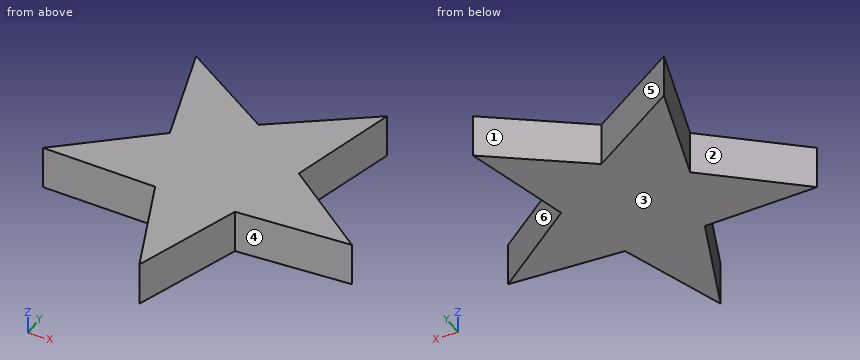
```python
from build123d import *

# Parameters (mm, degrees)
F1_DEPTH = 2


with BuildPart() as f1:
    # F0 (on Top) → F1 (new body)
    with BuildSketch(Plane.XY):
        Polygon((-2.938926, 0.954915), (0, 3.09017), (-4.349611, 5.986726), align=None)
        Polygon((4.349611, 5.986726), (0, 3.09017), (2.938926, 0.954915), align=None)
        Polygon((2.938926, 0.954915), (0, 3.09017), (-2.938926, 0.954915), (-1.816356, -2.5), (0, -2.5), (1.816356, -2.5), align=None)
        Polygon((-1.816356, -2.5), (-2.938926, 0.954915), (-7.037818, -2.286726), align=None)
        Polygon((0, -2.5), (-1.816356, -2.5), (0, -7.4), align=None)
        Polygon((7.037818, -2.286726), (2.938926, 0.954915), (1.816356, -2.5), align=None)
        Polygon((0, -7.4), (1.816356, -2.5), (0, -2.5), align=None)
    extrude(amount=F1_DEPTH)


solid = f1.part
```
Work out the finished part from the listing and answer in its coordinate system (mm). Face numbers are marked on the shaded views. A direction names the side the tool comes from. Coordinates: 2 decimals unless noted, no trailing zeros. Loops run counter-clockwise (first coordinate to the right, second up) from the corner with the lowest first, then second, coordinate; pieces in that order, holes last. Notation, with made-up numbers: M 34,-26 L 51,-26 A26 ccw 51,2 Z; hole C -2,37 d2. An arc over 180 degrees is marked long. Use CSV: the item, a comma, the result in double quotes. Start each with the question number.
(1) Find section B-B, the plane z = 1.35. Give the vertices of the cut face in (x, y), then the cut area to 3 significant figures.
(2) For a pull along X with two mould halves and no side action, classify the marked faces 1, 2 and 3 as +X half, -X half, draft (parallel to the pull), parting line (faces both ways), or undercut.
(3) Find section A-A, the plane x = -3.75. Give the vertices of the cut face in (y, z), then the cut area to 3 significant figures.
(4) For the marked faces 4, 5 and 6, determine the directions among +Z, -Z, +X, -X, +Y, -Y from which every point of the face is accessible in a straight line to the end or side of a thin tool.
(5) Given pin 1 Ø1 at (x, z) = (-3, 1) entering from -Y, flat-ended and moving along its own axis, determine where the tip first touches the part or whether it passes through.
(6) Consider line 1 (X direction, y = 4.5, z = 1.35); line 2 (X direction, y = 0.5, z = 1.75); line 3 (X direction, y = 2.75, z = 0.1). Determine where each line is inside the solid, lowest interval first.
(7) Find section D-D, the plane x = -0.25. Give the vertices of the cut face in (y, z), then the cut area to 3 significant figures.
(8) Find section C-C, the plane y = -0.5. Give the vertices of the cut face in (x, z), then the cut area to 3 significant figures.
Recorded:
1,outline,"M -7.04,-2.29 L -1.82,-2.5 L 0,-7.4 L 1.82,-2.5 L 7.04,-2.29 L 2.94,0.95 L 4.35,5.99 L 0,3.09 L -4.35,5.99 L -2.94,0.95 Z"
1,area,"67.2 mm^2"
2,face 1,"undercut"
2,face 2,"-X half"
2,face 3,"draft"
3,outline,"M -2.42,0 L 0.31,0 L 0.31,2 L -2.42,2 Z; M 3.85,0 L 5.59,0 L 5.59,2 L 3.85,2 Z"
3,area,"8.95 mm^2"
4,face 4,"+Z, -Z, +X, -Y"
4,face 5,"+Z, -Z, +Y"
4,face 6,"+Z, -Z, +X"
5,pin 1,"stops at y = -2.47"
6,line 1,"x = -3.93 to -2.12, 2.12 to 3.93"
6,line 2,"x = -3.51 to 3.51"
6,line 3,"x = -3.44 to 3.44"
7,outline,"M -6.73,0 L 3.26,0 L 3.26,2 L -6.73,2 Z"
7,area,"20.0 mm^2"
8,outline,"M -4.78,0 L 4.78,0 L 4.78,2 L -4.78,2 Z"
8,area,"19.1 mm^2"
